Autodesk Inventor part; units mm, degrees
ref_plane "YZ Plane" through (0, 0, 0) normal (1, 0, 0) x (0, 1, 0)
ref_plane "XZ Plane" through (0, 0, 0) normal (0, 1, 0) x (-1, 0, 0)
ref_plane "XY Plane" through (0, 0, 0) normal (0, 0, 1) x (1, 0, 0)
sketch "Sketch3" plane through (0, 0, 0) normal (0, 0, 1) x (1, 0, 0)
  circle A0 centre (46.0375, -6) radius 3.35
  circle A1 centre (46.0375, -67.15) radius 3.35
  circle A2 centre (5.6371, -75.5294) radius 3.35
  circle A3 centre (-30.1464, -57.7223) radius 3.35
  circle A4 centre (-24.2686, -18.1875) radius 3.35
  line L0 (152.6937, 0) -> (152.6937, -73.15) construction
  line L1 (0, 0) -> (152.6937, 0)
  arc A5 (0, 0) -> (28.1723, -73.15) centre (0, -42) ccw
  line L2 (152.6937, -73.15) -> (28.1723, -73.15)
  arc A6 (24.0029, -27.5826) -> (10.7567, -16.1486) centre (0, -42) ccw
  circle A7 centre (0, -42) radius 14.224
  line L3 (9.525, -14) -> (9.525, -14.3021)
  arc A8 (11.525, -12) -> (9.525, -14) centre (11.525, -14) ccw
  arc A9 (9.525, -14.3021) -> (10.7567, -16.1486) centre (11.525, -14.3021) ccw
  arc A10 (24.0029, -27.5826) -> (25.7174, -28.5528) centre (25.7174, -26.5528) ccw
  line L4 (152.6937, -73.15) -> (277.2151, -73.15)
  line L5 (305.3873, 0) -> (152.6937, 0)
  circle A11 centre (259.3498, -6) radius 3.35
  circle A12 centre (259.3498, -67.15) radius 3.35
  circle A13 centre (299.7503, -75.5294) radius 3.35
  circle A14 centre (335.5338, -57.7223) radius 3.35
  circle A15 centre (329.6559, -18.1875) radius 3.35
  arc A16 (277.2151, -73.15) -> (305.3873, 0) centre (305.3873, -42) ccw
  arc A17 (294.6307, -16.1486) -> (281.3845, -27.5826) centre (305.3873, -42) ccw
  circle A18 centre (305.3873, -42) radius 14.224
  line L6 (295.8623, -14) -> (295.8623, -14.3021)
  arc A19 (295.8623, -14) -> (293.8623, -12) centre (293.8623, -14) ccw
  arc A20 (294.6307, -16.1486) -> (295.8623, -14.3021) centre (293.8623, -14.3021) ccw
  arc A21 (279.67, -28.5528) -> (281.3845, -27.5826) centre (279.67, -26.5528) ccw
  line L7 (34.2736, -42.1004) -> (70.2455, -42.1004) construction
  line L8 (34.2736, -49.1004) -> (70.2455, -49.1004)
  line L9 (70.2455, -35.1004) -> (34.2736, -35.1004)
  arc A22 (34.2736, -35.1004) -> (34.2736, -49.1004) centre (34.2736, -42.1004) ccw
  arc A23 (70.2455, -49.1004) -> (70.2455, -35.1004) centre (70.2455, -42.1004) ccw
  line L10 (271.1137, -42.1004) -> (235.1419, -42.1004) construction
  line L11 (271.1137, -49.1004) -> (235.1419, -49.1004)
  line L12 (235.1419, -35.1004) -> (271.1137, -35.1004)
  arc A24 (271.1137, -49.1004) -> (271.1137, -35.1004) centre (271.1137, -42.1004) ccw
  arc A25 (235.1419, -35.1004) -> (235.1419, -49.1004) centre (235.1419, -42.1004) ccw
  circle A26 centre (103.364, -67.15) radius 3.35
  circle A27 centre (202.0233, -67.15) radius 3.35
  circle A28 centre (202.0233, -6) radius 3.35
  circle A29 centre (103.364, -6) radius 3.35
  line L13 (123.1183, -11.9896) -> (152.6937, -11.9896)
  line L14 (152.6937, -11.9896) -> (152.6937, -48.232) construction
  line L15 (152.6937, -48.232) -> (123.1183, -48.232)
  line L16 (121.1183, -46.232) -> (121.1183, -13.9896)
  arc A30 (123.1183, -11.9896) -> (121.1183, -13.9896) centre (123.1183, -13.9896) ccw
  arc A31 (121.1183, -46.232) -> (123.1183, -48.232) centre (123.1183, -46.232) ccw
  line L17 (182.269, -11.9896) -> (152.6937, -11.9896)
  line L18 (152.6937, -48.232) -> (182.269, -48.232)
  line L19 (184.269, -46.232) -> (184.269, -13.9896)
  arc A32 (184.269, -13.9896) -> (182.269, -11.9896) centre (182.269, -13.9896) ccw
  arc A33 (182.269, -48.232) -> (184.269, -46.232) centre (182.269, -46.232) ccw
  point P0 (24.5596, -28.5528)
  point P1 (9.525, -15.6699)
  point P2 (280.8278, -28.5528)
  point P3 (295.8623, -15.6699)
  point P4 (52.2596, -42.1004)
  point P5 (253.1278, -42.1004)
  dimension "d38" = 28.448
  dimension "d39" = 2
  dimension "d40" = 2
  dimension "d43" = 14
  dimension "d44" = 2
  dimension "d45" = 6
  dimension "d46" = 213.3123
extrude "Extrusion2" add sketch "Sketch3" along normal blind 3.175
properties part number "Mech Panel v7 skin exterior" material "Polycarbonate, Clear"
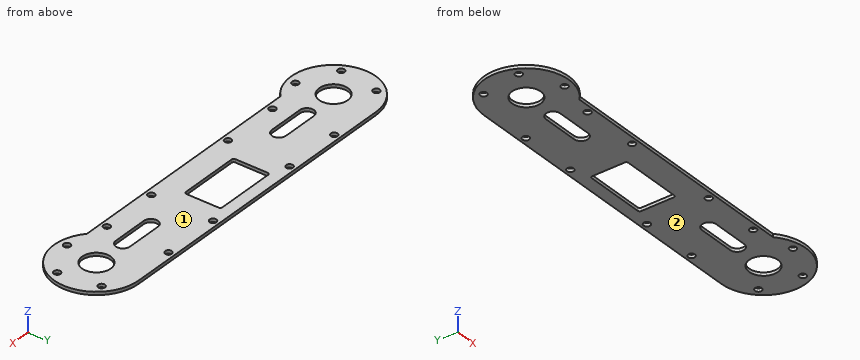
Work out the finished part from the listing and answer in its coordinate system (mm). Face numbers are marked on the shaded views. Coordinates: 2 decimals unless noted, no trailing zeros. Loops run counter-clockwise (first coordinate to the right, second up) from the corner with the lowest first, then second, coordinate; pieces in that order, holes last.
1) For a pull along Z with two mould halves and no side action, classify the marked faces 1 and 2 as +Z half, -Z half, draft (parallel to the pull), parting line (faces both ways), or undercut.
Results:
face 1: +Z half
face 2: -Z half
2) Section A-A (x = 132.5) is taken. Give the vertices of the cut face in (y, z) (3 decimals), plus the area to 3 significant figures.
Results:
outline: (-73.15, 0) - (-48.232, 0) - (-48.232, 3.175) - (-73.15, 3.175) - close; (-11.99, 0) - (0, 0) - (0, 3.175) - (-11.99, 3.175) - close
area: 117 mm2
3) Section C-C (x = 202) is taken. Give the vertices of the cut face in (y, z) (3 decimals), plus the area to 3 significant figures.
Results:
outline: (-73.15, 0) - (-70.5, 0) - (-70.5, 3.175) - (-73.15, 3.175) - close; (-63.8, 0) - (-9.35, 0) - (-9.35, 3.175) - (-63.8, 3.175) - close; (-2.65, 0) - (0, 0) - (0, 3.175) - (-2.65, 3.175) - close
area: 190 mm2
4) Section D-D (y = -42) is taken. Give the vertices of the cut face in (x, z) (3 decimals), plus the area to 3 significant figures.
Results:
outline: (-42, 0) - (-14.224, 0) - (-14.224, 3.175) - (-42, 3.175) - close; (14.224, 0) - (27.274, 0) - (27.274, 3.175) - (14.224, 3.175) - close; (77.245, 0) - (121.118, 0) - (121.118, 3.175) - (77.245, 3.175) - close; (184.269, 0) - (228.143, 0) - (228.143, 3.175) - (184.269, 3.175) - close; (278.113, 0) - (291.163, 0) - (291.163, 3.175) - (278.113, 3.175) - close; (319.611, 0) - (347.387, 0) - (347.387, 3.175) - (319.611, 3.175) - close
area: 538 mm2
5) Consider probe 1 along Y at (x, z) = (133, 2.7); probe 2 along Y at (x, z) = (306.5, 1.75); probe 3 along Y at (x, z) = (259.5, 2.5). Determine where each line is inside the solid, lowest interval first.
Results:
probe 1: y = -73.15 to -48.23, -11.99 to 0
probe 2: y = -83.99 to -56.18, -27.82 to -0.01
probe 3: y = -73.15 to -70.5, -63.8 to -49.1, -35.1 to -9.35, -2.65 to 0
6) Flat-ended cylindrical pins translate along their axes: pin 1 (1.5 mm diameter, centred on x = 254.5, z = 1.5, fed in from -Y); pin 2 (1.6 mm diameter, centred on y = -25.5, z = 2, fed in from +X); pin 3 (6 mm diameter, centred on x = -30.15, y = -57.72, fed in from +Z); pin 4 (1 mm diameter, centred on y = -17, z = 0.5, fed in from -X). Find the tip coordinate at first contact, or state that the pin passes through.
Results:
pin 1: stops at y = -73.15
pin 2: stops at x = 344.34
pin 3: passes through
pin 4: stops at x = -34.11
7) Section B-B (y = -6) is taken. Give the vertices of the cut face in (x, z) (1 decimal), plus the area to 3 significant figures.
Results:
outline: (-21.6, 0) - (42.7, 0) - (42.7, 3.2) - (-21.6, 3.2) - close; (49.4, 0) - (100, 0) - (100, 3.2) - (49.4, 3.2) - close; (106.7, 0) - (198.7, 0) - (198.7, 3.2) - (106.7, 3.2) - close; (205.4, 0) - (256, 0) - (256, 3.2) - (205.4, 3.2) - close; (262.7, 0) - (327, 0) - (327, 3.2) - (262.7, 3.2) - close
area: 1,020 mm2
